Geometry check sheet. Reference: the model listing, model coordinates, mm. A direction names the side the tool comes from. Coordinates: 2 decimals unless noted, no trailing zeros. Order: outer loops, then holes, each group sorted by start corner. A loop starts at its lowest first (then second) coordinate and runs counter-clockwise, first axis right, second up. Notation, with made-up numbers: (19.5, 64) - (27.5, 64) arc R19 cw to (27.5, 68) - close; hole circle Ø1 at (-4, 43). An arc over 180 degrees is marked (long way). Return JSON: item names as keys, results as strings. Group by question number.
Item 1: Section check C-C on z = 20. Enter the section's corners in (x, y), then the cut area to 3 significant figures.
Item 2: Section check A-A on x = 216. Enter the section's corners in (y, z), then the cut area to 3 significant figures.
Item 3: Gauge pin test, flat ends, axial feed: pin 1 (12 mm diameter, centred on x = 674.11, y = 25.4, fed in from +Z); pin 2 (1.5 mm diameter, centred on y = 19, z = 8.5, fed in from -X). Record the tip position at first contact, or that the pin passes through.
Item 4: Section check B-B on y = 72.5. Enter the section's corners in (x, z).
Item 5: Draft check along Z on faces 3 (the flat face through (339, 77, 6)), 4 (the flat face through (339, 153, 20)), 5 (the flat face through (339, 78, 0)), 6 (the flat face through (339, 77, 51.46)). Enter one of: pulls with the +Z half, pulls with the -Z half, needs draft (parallel to the pull), parting line crosses it, or undercut.
Item 6: Scan lines: probe 1 along Y at (x, z) = (674.11, 4.3); probe 2 along Z at (x, y) = (291, 17); probe 3 along Z at (x, y) = (382, 15). Record each from-to range of solid material in increasing order.
Item 7: Tool access check on faces 1 (the flat face through (3.791, 70.476, 4.645)), 2 (the flat face through (339, 6, 21)). Record the directions out of +Z, -Z, +X, -X, +Y, -Y that give a thin tool (end or side, any length) a straight path to the whole face; none if there is none.
from build123d import *

# Parameters (mm, degrees)
SKETCH1_W           = 686.81
SKETCH1_H           = 153
BOSS_EXTRUDE1_DEPTH = 51.46
CUT_EXTRUDE1_DEPTH  = 153
SHELL1_T            = -6
SKETCH3_R           = 3.75
CUT_EXTRUDE2_DEPTH  = 6
FILLET1_R           = 10


with BuildPart() as part:
    # Sketch1 → Boss-Extrude1 (new body)
    with BuildSketch(Plane.XY):
        with Locations((343.405, 76.5)):
            Rectangle(SKETCH1_W, SKETCH1_H)
    extrude(amount=BOSS_EXTRUDE1_DEPTH)

    # Sketch2 → Cut-Extrude1 (cut)
    with BuildSketch(Plane.XZ):
        Polygon((0, 0), (42, 51.46), (-52.578690856, 191.351676445), (-175.691026148, 25.73), align=None)
        Polygon((686.81, 0), (644.81, 51.46), (843.619472118, 127.98285715), align=None)
    extrude(amount=-CUT_EXTRUDE1_DEPTH, mode=Mode.SUBTRACT)

    # Shell1
    shell1_openings = [part.faces().sort_by_distance(p)[0] for p in [
        (21, 76.5, 25.73),
        (665.81, 76.5, 25.73),
    ]]
    offset(amount=SHELL1_T, openings=shell1_openings, kind=Kind.INTERSECTION)

    # Sketch3 → Cut-Extrude2 (cut)
    with BuildSketch(Plane.XY.offset(6)):
        with Locations((12.7, 25.4)):
            Circle(SKETCH3_R)
        with Locations((12.7, 127.6)):
            Circle(SKETCH3_R)
        with Locations((674.11, 25.4)):
            Circle(SKETCH3_R)
        with Locations((674.11, 127.6)):
            Circle(SKETCH3_R)
    extrude(amount=-CUT_EXTRUDE2_DEPTH, mode=Mode.SUBTRACT)

    # Fillet1
    fillet1_edges = [part.edges().sort_by_distance(p)[0] for p in [
        (343.405, 0, 51.46),
        (343.405, 153, 51.46),
        (343.405, 6, 45.46),
        (343.405, 147, 45.46),
    ]]
    fillet(fillet1_edges, radius=FILLET1_R)


solid = part.part
Computed:
{
 "1": {"outline": "(16.32, 0) - (670.49, 0) - (670.49, 6) - (16.32, 6) - close; (16.32, 147) - (670.49, 147) - (670.49, 153) - (16.32, 153) - close", "area": "7,850 mm²"},
 "2": {"outline": "(0, 0) - (153, 0) - (153, 41.46) arc R10 ccw to (143, 51.46) - (10, 51.46) arc R10 ccw to (0, 41.46) - close; hole (6, 6) - (147, 6) - (147, 35.46) arc R10 ccw to (137, 45.46) - (16, 45.46) arc R10 ccw to (6, 35.46) - close", "area": "2,310 mm²"},
 "3": {"pin 1": "stops at z = 6", "pin 2": "passes through"},
 "4": {"outline": "(0, 0) - (686.81, 0) - (681.91, 6) - (4.9, 6) - close; (37.1, 45.46) - (649.71, 45.46) - (644.81, 51.46) - (42, 51.46) - close"},
 "5": {"face 3": "undercut", "face 4": "needs draft", "face 5": "pulls with the -Z half", "face 6": "pulls with the +Z half"},
 "6": {"probe 1": "y = 0 to 21.65, 29.15 to 123.85, 131.35 to 153", "probe 2": "z = 0 to 6, 45.46 to 51.46", "probe 3": "z = 0 to 6, 45.41 to 51.46"},
 "7": {"face 1": "+Z, -X, +Y, -Y", "face 2": "+X, -X"}
}
